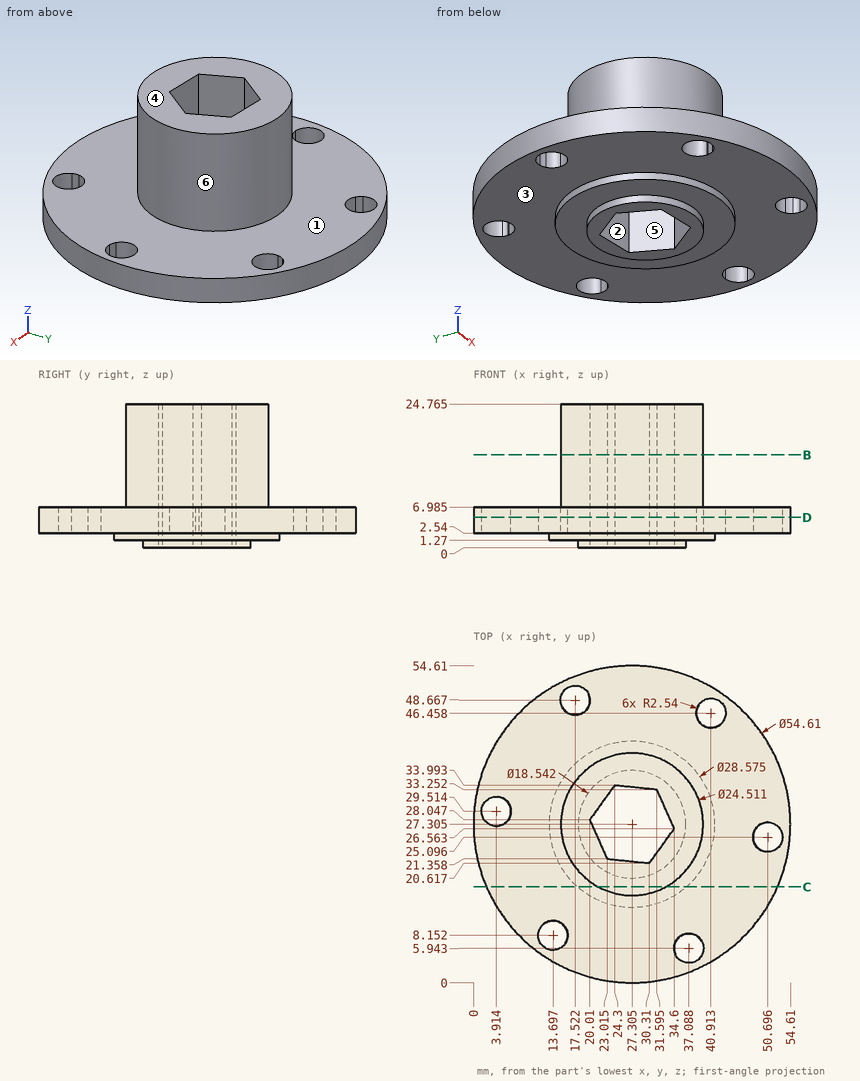
Here's the drawing with two shaded views (mm, measured from the low corner). I have some questions. A direction names the side the tool comes from. Give positions to 0.01 mm unless a question says otherwise; leave off trailing zeros. Order: outer loops, then holes, each group sorted by start corner. A loop starts at its lowest first (then second) coordinate and runs counter-clockwise, first axis right, second up.
Q1. I'm going to push flat-ended pins straight in: P1, Ø12, axis at x = 42.5, y = 9, coming from the -Z side; P2, Ø10, axis at x = 16.5, z = 7.5, coming from the +Y side; P3, Ø12, axis at x = 40.5, y = 44.5, coming from the +Z side (3 decimals). Where does each tip first touch, or does it pass through?
Q2. For the marked faces 1, 2 and 3, which set-ups out of +Z, -Z, +X, -X, +Y, -Y let a thin tool reach every point of the face, with its end or its side?
Q3. We'd pull the mould along Y, two halves only. Please class the marked faces 4, 5 and 6: +Y half, -Y half, draft (parallel to the pull), parting line (faces both ways), or undercut.
Q4. Suppose I cut it at B-B, the plane z = 16. Write out the boundary of the cut face in (x, y) (1 decimal), and give its area (3 significant figures).
Q5. Suppose I cut it at C-C, the plane y = 16.5. Write out the boundary of the cut face in (x, z) (1 decimal), and give its area (3 significant figures).
Q6. Suppose I cut it at D-D, the plane z = 5.25. Write out the boundary of the cut face in (x, y) (1 decimal).
Q7. If I drill on line 1 along Z through (x, y) = (20, 37) (1 decimal); line 2 along Z through (x, y) = (34.5, 13.5) (1 decimal); line 3 along Y through (x, z) = (30.5, 23.5) (1 decimal), over which ranges is the centre line in solid material (lowest first)?
Solution:
1. P1: stops at z = 2.54
1. P2: stops at y = 53.98
1. P3: stops at z = 6.985
2. face 1: +Z
2. face 2: +Z, -Z
2. face 3: -Z
3. face 4: draft
3. face 5: undercut
3. face 6: parting line
4. outline: circle Ø24.5 at (27.3, 27.3); hole (20, 28) - (23, 21.4) - (30.3, 20.6) - (34.6, 26.6) - (31.6, 33.3) - (24.3, 34) - close
4. area: 332 mm2
5. outline: (2.2, 2.5) - (18, 2.5) - (18, 1.3) - (36.7, 1.3) - (36.7, 2.5) - (52.4, 2.5) - (52.4, 7) - (33.1, 7) - (33.1, 24.8) - (21.5, 24.8) - (21.5, 7) - (2.2, 7) - close
5. area: 452 mm2
6. outline: circle Ø54.6 at (27.3, 27.3); hole circle Ø5.1 at (3.9, 29.5); hole circle Ø5.1 at (13.7, 8.2); hole circle Ø5.1 at (17.5, 48.7); hole (20, 28) - (23, 21.4) - (30.3, 20.6) - (34.6, 26.6) - (31.6, 33.3) - (24.3, 34) - close; hole circle Ø5.1 at (37.1, 5.9); hole circle Ø5.1 at (40.9, 46.5); hole circle Ø5.1 at (50.7, 25.1)
7. line 1: z = 1.3 to 24.8
7. line 2: z = 2.5 to 7
7. line 3: y = 15.5 to 20.9, 33.4 to 39.1
